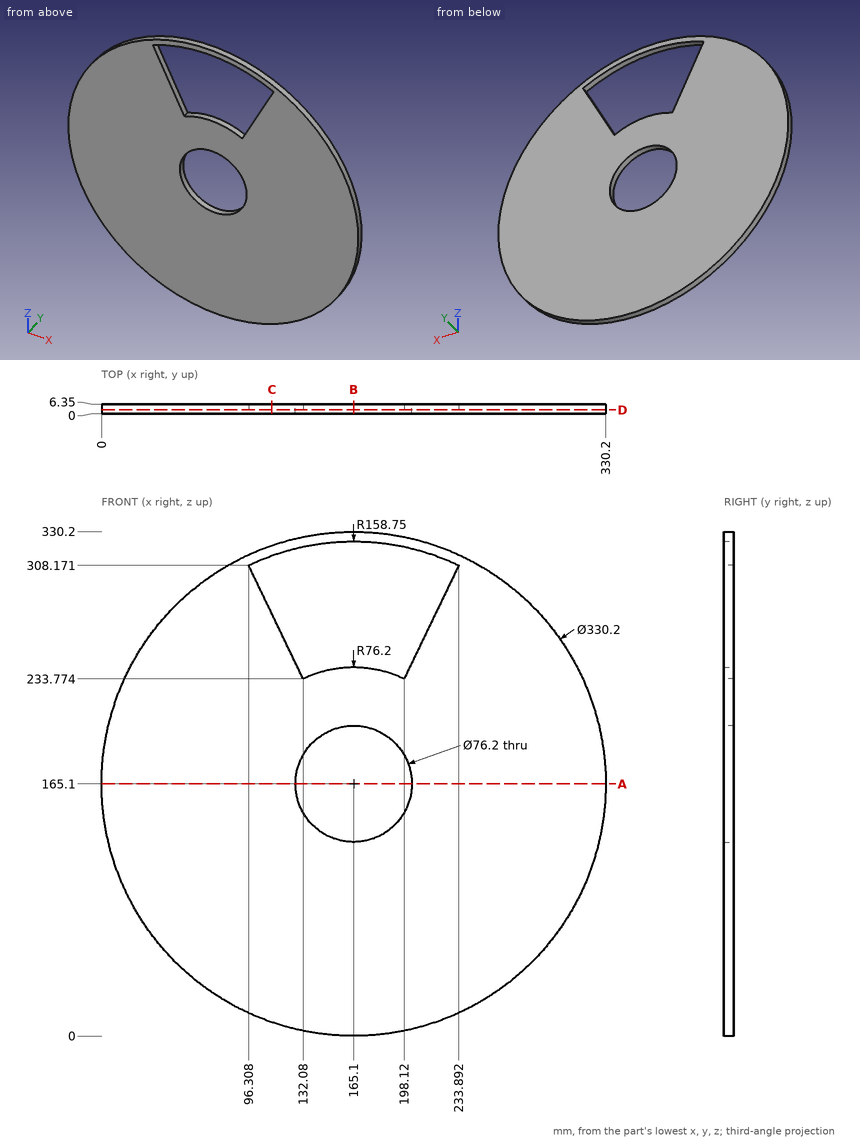
Job drawing, mm, ordinate dimensions from the low corner. One solid piece. Give positions to 0.01 mm unless a question says otherwise; leave off trailing zeros. Order: outer loops, then holes, each group sorted by start corner. A loop starts at its lowest first (then second) coordinate and runs counter-clockwise, first axis right, second up. Notation, with made-up numbers: M -18.75,87 L 23.25,87 A16 ccw 23.25,97 Z; hole C 84,-14 d1. An arc over 180 degrees is marked long. Put each result on its own line as item: value. Start each with the question number.
(1) Pin check, flat tips, straight feed: pin 1 Ø1.5 at (y, z) = (0.5, 119) entering from +X; pin 2 Ø3 at (x, y) = (38, 1.5) entering from -Z; pin 3 Ø2 at (y, z) = (3.5, 79.5) entering from +X. Stop position of each tip, or through.
(2) Band-saw the part on D-D on y = 2.5. Give the cut face in (x, z).
(3) Band-saw the part on C-C on x = 111.5. Give the cut face in (y, z), then the cut area to 3 significant figures.
(4) Band-saw the part on B-B on x = 165.1. Give the cut face in (y, z).
(5) Drill centre lines: L1, parallel to X at y = 4.25, z = 165.1; L2, parallel to Z at x = 185, y = 5.25 (1 decimal); L3, parallel to X at y = 1.75, z = 119.5. Where is each one in solid material? Low to high. Write a range as [from, to].
(6) Band-saw the part on A-A on z = 165.1. Give the cut face in (x, y).
Results below:
1. pin 1: stops at x = 323.85
1. pin 2: stops at z = 57.94
1. pin 3: stops at x = 306.88
2. outline: C 165.1,165.1 d330.2; hole M 96.31,308.17 L 132.08,233.77 A76.2 cw 198.12,233.77 L 233.89,308.17 A158.75 ccw Z; hole C 165.1,165.1 d76.2
3. outline: M 0,8.94 L 6.35,8.94 L 6.35,276.58 L 0,276.58 Z; M 0,314.53 L 6.35,314.53 L 6.35,321.26 L 0,321.26 Z
3. area: 1,740 mm2
4. outline: M 0,0 L 6.35,0 L 6.35,127 L 0,127 Z; M 0,203.2 L 6.35,203.2 L 6.35,241.3 L 0,241.3 Z; M 0,323.85 L 6.35,323.85 L 6.35,330.2 L 0,330.2 Z
5. L1: x = [0, 127], [203.2, 330.2]
5. L2: z = [1.2, 132.6], [197.6, 238.7], [322.6, 329]
5. L3: x = [6.42, 323.78]
6. outline: M 0,0 L 127,0 L 127,6.35 L 0,6.35 Z; M 203.2,0 L 330.2,0 L 330.2,6.35 L 203.2,6.35 Z
